from build123d import *

# Parameters (mm, degrees)
CUT_EXTRUDE_1_DEPTH = 2
FILLET_1_R          = 0.3
CHAMFER_1_SIZE      = 0.3


with BuildPart() as part:
    # Эскиз1 → Повернуть1 (revolve)
    with BuildSketch(Plane(origin=(0, 0, 0), x_dir=(0, 0, -1), z_dir=(1, 0, 0))):
        Polygon((0, 0), (0, 3.5), (4, 3.5), (4, 2), (16, 2), (16, 0), align=None)
    revolve(axis=Axis((0, 0, 0), (0, 0, 1)))

    # Эскиз2 → Вырез-Вытянуть1 (cut)
    with BuildSketch(Plane.XY):
        Polygon((1.732050808, 0), (0.866025404, 1.5), (-0.866025404, 1.5), (-1.732050808, 0), (-0.866025404, -1.5), (0.866025404, -1.5), align=None)
    extrude(amount=-CUT_EXTRUDE_1_DEPTH, mode=Mode.SUBTRACT)

    # Скругление1
    fillet_1_edges = [part.edges().sort_by_distance(p)[0] for p in [
        (0, -2, -4),
    ]]
    fillet(fillet_1_edges, radius=FILLET_1_R)

    # Фаска1
    chamfer_1_edges = [part.edges().sort_by_distance(p)[0] for p in [
        (0, -2, -16),
    ]]
    chamfer(chamfer_1_edges, length=CHAMFER_1_SIZE)


solid = part.part
The listing builds one solid part. Answer for the finished solid, in the listing's coordinates (mm). A direction names the side the tool comes from. Give positions to 0.01 mm unless a question says otherwise; leave off trailing zeros. Order: outer loops, then holes, each group sorted by start corner. A loop starts at its lowest first (then second) coordinate and runs counter-clockwise, first axis right, second up. Notation, with made-up numbers: (33.25, 20.25) - (64.25, 20.25) arc R38 ccw to (64.25, 58.25) - close; hole circle Ø5 at (-25.5, 76.5). An arc over 180 degrees is marked (long way). One line per item, written item: value. Start each with the question number.
1) Find the intervals of material crossed by L1, parallel to Z at x = 2, y = 2.25; L2, parallel to Y at x = 1, z = -11.5, in increasing order.
2) A cutting plane is placed at C-C on z = -7.75. Give the vertices of the cut face in (x, y), then the cut area to 3 significant figures.
3) A cutting plane is placed at A-A on z = -0.75. Give the vertices of the cut face in (x, y), then the cut area to 3 significant figures.
4) A cutting plane is placed at B-B on x = 0. Give the vertices of the cut face in (y, z), then the cut area to 3 significant figures.
5) The mould has two halves that part along Y. Classify faces 1 (the face through (1.341, 3.233, -2.028)), 2 (the face through (0, -2, 0)), 3 (the face through (1.305, 0.74, -0.986)): released by +Y, released by -Y, zero draft, split by the parting line, or undercut.
6) A cutting plane is placed at D-D on z = -2.5. Give the vertices of the cut face in (x, y).
7) Given pin 1 Ø2 at (x, z) = (-0.5, -14.5) entering from -Y; pin 2 Ø2 at (x, z) = (-2, -9) entering from +Y; pin 3 Ø1.5 at (x, z) = (2.5, -6.5) entering from +Y, each flat-ended and moving along its own axis, determine where each tip first touches the part or whether it passes through.
8) A tool of negligible diameter and unlimited length cuts with its end or side. For faces 4 (the face through (-1.305, -0.74, -0.986)), 5 (the face through (2, 0, -10)), 6 (the face through (0, 0, -16)), from which of +Z, -Z, +X, -X, +Y, -Y can it reach the whole face along a straight path? Write none if from no direction.
Answer sheet:
1. L1: z = -4 to 0
1. L2: y = -1.73 to 1.73
2. outline: circle Ø4 at (0, 0)
2. area: 12.6 mm2
3. outline: circle Ø7 at (0, 0); hole (-1.73, 0) - (-0.87, -1.5) - (0.87, -1.5) - (1.73, 0) - (0.87, 1.5) - (-0.87, 1.5) - close
3. area: 30.7 mm2
4. outline: (-3.5, -4) - (-2.3, -4) arc R0.3 cw to (-2, -4.3) - (-2, -15.7) - (-1.7, -16) - (1.7, -16) - (2, -15.7) - (2, -4.3) arc R0.3 cw to (2.3, -4) - (3.5, -4) - (3.5, 0) - (1.5, 0) - (1.5, -2) - (-1.5, -2) - (-1.5, 0) - (-3.5, 0) - close
4. area: 69.9 mm2
5. face 1: split by the parting line
5. face 2: zero draft
5. face 3: undercut
6. outline: circle Ø7 at (0, 0)
7. pin 1: stops at y = -2
7. pin 2: stops at y = 1.73
7. pin 3: stops at y = 0.97
8. face 4: +Z
8. face 5: -Z
8. face 6: -Z, +X, -X, +Y, -Y
